Could you check a few things on this model? Use its own coordinates, in mm. A direction names the side the tool comes from. Round coordinates to 2 decimals unless told otherwise and drop trailing zeros. Order: outer loops, then holes, each group sorted by start corner. A loop starts at its lowest first (then second) coordinate and runs counter-clockwise, first axis right, second up. Notation, with made-up numbers: (-29.75, 53) - (-23.75, 53) arc R10 cw to (-23.75, 68) - close; hole circle Ø1 at (-17.75, 88.5). An arc over 180 degrees is marked (long way). Return JSON: item names as keys, results as strings. Group by question number.
from build123d import *

# Parameters (mm, degrees)
SKETCH1_W               = 185
SKETCH1_H               = 100
BOSS_EXTRUDE1_DEPTH     = 16
CUT_EXTRUDE1_DEPTH      = 107.359061673
CUT_EXTRUDE1_DEPTH_BACK = 107.359061673
F_1_0MM_DOWEL_HOLE1_D   = 29.5
CHAMFER1_SIZE           = 3


with BuildPart() as part:
    # Sketch1 → Boss-Extrude1 (new body)
    with BuildSketch(Plane(origin=(0, 0, 0), x_dir=(1, 0, 0), z_dir=(0, 1, 0))):
        Rectangle(SKETCH1_W, SKETCH1_H)
    extrude(amount=BOSS_EXTRUDE1_DEPTH)

    # Sketch2 → Cut-Extrude1 (cut, two sides: drawn at the far end of the back side and taken through both)
    with BuildSketch(Plane(origin=(0, 16, 0), x_dir=(1, 0, 0), z_dir=(0, 1, 0)).offset(-CUT_EXTRUDE1_DEPTH_BACK)):
        with BuildLine():
            Line((-75.75, 39.25), (-49.25, 39.25))
            ThreePointArc((-49.25, 39.25), (-42.5, 32.5), (-49.25, 25.75))
            Line((-49.25, 25.75), (-75.75, 25.75))
            ThreePointArc((-75.75, 25.75), (-82.5, 32.5), (-75.75, 39.25))
        make_face()
        with BuildLine():
            Line((-49.25, -39.25), (-75.75, -39.25))
            ThreePointArc((-75.75, -39.25), (-82.5, -32.5), (-75.75, -25.75))
            Line((-75.75, -25.75), (-49.25, -25.75))
            ThreePointArc((-49.25, -25.75), (-42.5, -32.5), (-49.25, -39.25))
        make_face()
        with BuildLine():
            Line((49.25, 39.25), (75.75, 39.25))
            ThreePointArc((75.75, 39.25), (82.5, 32.5), (75.75, 25.75))
            Line((75.75, 25.75), (49.25, 25.75))
            ThreePointArc((49.25, 25.75), (42.5, 32.5), (49.25, 39.25))
        make_face()
        with BuildLine():
            Line((49.25, -25.75), (75.75, -25.75))
            ThreePointArc((75.75, -25.75), (82.5, -32.5), (75.75, -39.25))
            Line((75.75, -39.25), (49.25, -39.25))
            ThreePointArc((49.25, -39.25), (42.5, -32.5), (49.25, -25.75))
        make_face()
    extrude(amount=CUT_EXTRUDE1_DEPTH + CUT_EXTRUDE1_DEPTH_BACK, mode=Mode.SUBTRACT)

    # Ø1.0mm Dowel Hole1 (through all)
    with Locations(Plane(origin=(0, 16, 0), x_dir=(1, 0, 0), z_dir=(0, 1, 0))):
        with Locations((0, 0)):
            Hole(F_1_0MM_DOWEL_HOLE1_D / 2)

    # Chamfer1
    chamfer1_edges = [part.edges().sort_by_distance(p)[0] for p in [
        (14.75, 16, 0),
    ]]
    chamfer(chamfer1_edges, length=CHAMFER1_SIZE)


solid = part.part
1) I want a section at D-D, the plane x = 64. List the corners of the cut face in (y, z) for me.
2) For faces 5 (the flat face through (63, 8, 39.25)), 6 (the flat face through (-22, 16, -1)), which set-ups out of +Z, -Z, +X, -X, +Y, -Y let a thin tool reach every point of the face, with its end or its side?
3) If I drill on line 1 along Z through (x, y) = (-67, 4.75); line 2 along X through (y, z) = (13, 29); line 3 along Z through (x, y) = (0, 5), over which ranges is the centre line in solid material (lowest first)? Write a range as from..to.
4) I want a section at C-C, the plane y = 10.25. List the corners of the cut face in (x, z) for me, plus the area to 3 significant figures.
5) I want a section at A-A, the plane z = 32.5. List the corners of the cut face in (x, y) for me, plus the area to 3 significant figures.
6) I want a section at B-B, the plane x = 0. List the corners of the cut face in (y, z) for me.
7) We'd pull the mould along Z, two halves only. Please class faces 1 (the flat face through (-1, 8, 50)), 2 (the flat face through (-63, 8, -39.25)), 3 (the flat face through (-22, 0, -1)), 4 (the flat face through (62, 8, -39.25)): +Z half, -Z half, draft (parallel to the pull), parting line (faces both ways), or undercut.
Outcome:
{
 "1": {"outline": "(0, -50) - (16, -50) - (16, -39.25) - (0, -39.25) - close; (0, -25.75) - (16, -25.75) - (16, 25.75) - (0, 25.75) - close; (0, 39.25) - (16, 39.25) - (16, 50) - (0, 50) - close"},
 "2": {"face 5": "+Y, -Y", "face 6": "+Z, -Z, +X, -X, +Y"},
 "3": {"line 1": "-50..-39.25, -25.75..25.75, 39.25..50", "line 2": "-92.5..-81.52, -43.48..43.48, 81.52..92.5", "line 3": "-50..-14.75, 14.75..50"},
 "4": {"outline": "(-92.5, -50) - (92.5, -50) - (92.5, 50) - (-92.5, 50) - close; hole (-75.75, -39.25) - (-49.25, -39.25) arc R6.75 ccw to (-49.25, -25.75) - (-75.75, -25.75) arc R6.75 ccw to start; hole (-75.75, 25.75) - (-49.25, 25.75) arc R6.75 ccw to (-49.25, 39.25) - (-75.75, 39.25) arc R6.75 ccw to start; hole circle Ø29.5 at (0, 0); hole (49.25, -39.25) - (75.75, -39.25) arc R6.75 ccw to (75.75, -25.75) - (49.25, -25.75) arc R6.75 ccw to start; hole (49.25, 25.75) - (75.75, 25.75) arc R6.75 ccw to (75.75, 39.25) - (49.25, 39.25) arc R6.75 ccw to start", "area": "15,800 mm^2"},
 "5": {"outline": "(-92.5, 0) - (-82.5, 0) - (-82.5, 16) - (-92.5, 16) - close; (-42.5, 0) - (42.5, 0) - (42.5, 16) - (-42.5, 16) - close; (82.5, 0) - (92.5, 0) - (92.5, 16) - (82.5, 16) - close", "area": "1,680 mm^2"},
 "6": {"outline": "(0, -50) - (16, -50) - (16, -17.75) - (13, -14.75) - (0, -14.75) - close; (0, 14.75) - (13, 14.75) - (16, 17.75) - (16, 50) - (0, 50) - close"},
 "7": {"face 1": "+Z half", "face 2": "undercut", "face 3": "draft", "face 4": "undercut"}
}
